```python
from build123d import *

# Parameters (mm, degrees)
SKETCH1_W                                            = 15
SKETCH1_H                                            = 15
SKETCH1_W_2                                          = 4
SKETCH1_H_2                                          = 4
BOSS_EXTRUDE1_DEPTH                                  = 10
FILLET1_R                                            = 0.5
CBORE_FOR_M1_6_HEXAGON_SOCKET_HEAD_CAP_S_D           = 1.8
CBORE_FOR_M1_6_HEXAGON_SOCKET_HEAD_CAP_S_CBORE_D     = 3.3
CBORE_FOR_M1_6_HEXAGON_SOCKET_HEAD_CAP_S_CBORE_DEPTH = 1.8
M2_TAPPED_HOLE1_AT_2_COUNT                           = 2
M2_TAPPED_HOLE1_AT_2_PITCH                           = 9.5
CHAMFER1_SIZE                                        = 1
CUT_EXTRUDE1_DEPTH                                   = 2
M2_TAPPED_HOLE2_D                                    = 1.6
M2_TAPPED_HOLE2_DEPTH                                = 2
M2_TAPPED_HOLE2_TIP                                  = 0.480688495
SKETCH12_R                                           = 4.5
SKETCH12_R_2                                         = 3
CUT_EXTRUDE2_DEPTH                                   = 2
FILLET2_R                                            = 1
CHAMFER2_SIZE                                        = 1


with BuildPart() as part:
    # Sketch1 → Boss-Extrude1 (new body)
    with BuildSketch(Plane.XY):
        Rectangle(SKETCH1_W, SKETCH1_H)
        Rectangle(SKETCH1_W_2, SKETCH1_H_2, mode=Mode.SUBTRACT)
    extrude(amount=-BOSS_EXTRUDE1_DEPTH)

    # Fillet1
    fillet1_edges = [part.edges().sort_by_distance(p)[0] for p in [
        (2, 2, -5),
        (2, -2, -5),
        (-2, -2, -5),
        (-2, 2, -5),
    ]]
    fillet(fillet1_edges, radius=FILLET1_R)

    # CBORE for M1.6 Hexagon socket head cap screws1 (through all)
    with Locations(Plane(origin=(0, 7.5, 0), x_dir=(1, 0, 0), z_dir=(0, 1, 0))):
        with Locations((0, 5)):
            CounterBoreHole(CBORE_FOR_M1_6_HEXAGON_SOCKET_HEAD_CAP_S_D / 2, CBORE_FOR_M1_6_HEXAGON_SOCKET_HEAD_CAP_S_CBORE_D / 2, CBORE_FOR_M1_6_HEXAGON_SOCKET_HEAD_CAP_S_CBORE_DEPTH)

    # Sketch6 → M2 Tapped Hole1 (revolve, cut)
    with BuildSketch(Plane(origin=(-7.5, 5, -5), x_dir=(0, 0, 1), z_dir=(0, 1, 0))):
        Polygon((0, 0), (0, 5.480688495), (0.8, 5), (0.8, 0), align=None)
    m2_tapped_hole1 = revolve(axis=Axis((-13.85, 5, -5), (1, 0, 0)), mode=Mode.SUBTRACT)

    # M2 Tapped Hole1 at 2: M2 Tapped Hole1 ×2
    with Locations(*[(0, -i * M2_TAPPED_HOLE1_AT_2_PITCH, 0) for i in range(1, M2_TAPPED_HOLE1_AT_2_COUNT)]):
        add(m2_tapped_hole1, mode=Mode.SUBTRACT)

    # Mirror1: M2 Tapped Hole1 across plane
    add(m2_tapped_hole1.mirror(Plane(origin=(0, 0, 0), x_dir=(0, 0, 1), z_dir=(1, 0, 0))), mode=Mode.SUBTRACT)

    # Mirror1 copy 1 sketch → Mirror1 copy 1 (revolve, cut)
    with BuildSketch(Plane(origin=(7.5, -4.5, -5), x_dir=(0, 0, 1), z_dir=(0, 1, 0))):
        Polygon((0, 0), (0, -5.480688495), (0.8, -5), (0.8, 0), align=None)
    revolve(axis=Axis((13.85, -4.5, -5), (1, 0, 0)), mode=Mode.SUBTRACT)

    # Chamfer1
    chamfer1_edges = [part.edges().sort_by_distance(p)[0] for p in [
        (7.5, -7.5, -5),
        (-7.5, -7.5, -5),
    ]]
    chamfer(chamfer1_edges, length=CHAMFER1_SIZE)

    # Sketch8 → Cut-Extrude1 (cut)
    with BuildSketch(Plane(origin=(0, 0, -10), x_dir=(-1, 0, 0), z_dir=(0, 0, -1))):
        with BuildLine():
            ThreePointArc((-5.49078868, 5.818181818), (-5.656854249, 5.656854249), (-5.818181818, 5.49078868))
            ThreePointArc((-5.818181818, 5.49078868), (-5.715871463, 1.956735399), (-2.181818182, 2.059045755))
            ThreePointArc((-2.181818182, 2.059045755), (-2.121320344, 2.121320344), (-2.059045755, 2.181818182))
            ThreePointArc((-2.059045755, 2.181818182), (-1.956735399, 5.715871463), (-5.49078868, 5.818181818))
        make_face()
        with BuildLine():
            ThreePointArc((-5.49078868, -5.818181818), (-5.656854249, -5.656854249), (-5.818181818, -5.49078868))
            ThreePointArc((-5.818181818, -5.49078868), (-5.715871463, -1.956735399), (-2.181818182, -2.059045755))
            ThreePointArc((-2.181818182, -2.059045755), (-2.121320344, -2.121320344), (-2.059045755, -2.181818182))
            ThreePointArc((-2.059045755, -2.181818182), (-1.956735399, -5.715871463), (-5.49078868, -5.818181818))
        make_face()
        with BuildLine():
            ThreePointArc((5.49078868, 5.818181818), (5.656854249, 5.656854249), (5.818181818, 5.49078868))
            ThreePointArc((5.818181818, 5.49078868), (5.715871463, 1.956735399), (2.181818182, 2.059045755))
            ThreePointArc((2.181818182, 2.059045755), (2.121320344, 2.121320344), (2.059045755, 2.181818182))
            ThreePointArc((2.059045755, 2.181818182), (1.956735399, 5.715871463), (5.49078868, 5.818181818))
        make_face()
        with BuildLine():
            ThreePointArc((5.49078868, -5.818181818), (5.656854249, -5.656854249), (5.818181818, -5.49078868))
            ThreePointArc((5.818181818, -5.49078868), (5.715871463, -1.956735399), (2.181818182, -2.059045755))
            ThreePointArc((2.181818182, -2.059045755), (2.121320344, -2.121320344), (2.059045755, -2.181818182))
            ThreePointArc((2.059045755, -2.181818182), (1.956735399, -5.715871463), (5.49078868, -5.818181818))
        make_face()
    extrude(amount=-CUT_EXTRUDE1_DEPTH, mode=Mode.SUBTRACT)

    # M2 Tapped Hole2
    with Locations(Plane(origin=(0, 0, -10), x_dir=(-1, 0, 0), z_dir=(0, 0, -1))):
        with Locations((-6, 0), (0, 6), (6, 0), (0, -6)):
            Hole(M2_TAPPED_HOLE2_D / 2, depth=M2_TAPPED_HOLE2_DEPTH)
            with Locations((0, 0, -(M2_TAPPED_HOLE2_DEPTH + M2_TAPPED_HOLE2_TIP / 2))):  # 118° drill point
                Cone(0, M2_TAPPED_HOLE2_D / 2, M2_TAPPED_HOLE2_TIP, mode=Mode.SUBTRACT)

    # Sketch12 → Cut-Extrude2 (cut)
    with BuildSketch(Plane(origin=(0, 0, -10), x_dir=(-1, 0, 0), z_dir=(0, 0, -1))):
        Circle(SKETCH12_R)
        with Locations(Location((0, 0, 0), (0, 0, 180))):
            Circle(SKETCH12_R_2, mode=Mode.SUBTRACT)
    extrude(amount=-CUT_EXTRUDE2_DEPTH, mode=Mode.SUBTRACT)

    # Fillet2
    fillet2_edges = [part.edges().sort_by_distance(p)[0] for p in [
        (1.294196531, 4.309878808, -9),
        (-1.294196531, 4.309878808, -9),
        (4.309878808, 1.294196531, -9),
        (4.309878808, -1.294196531, -9),
        (-1.294196531, -4.309878808, -9),
        (1.294196531, -4.309878808, -9),
        (-4.309878808, -1.294196531, -9),
        (-4.309878808, 1.294196531, -9),
    ]]
    fillet(fillet2_edges, radius=FILLET2_R)

    # Chamfer2
    chamfer2_edges = [part.edges().sort_by_distance(p)[0] for p in [
        (-7.5, 7.5, -5),
        (7.5, 7.5, -5),
    ]]
    chamfer(chamfer2_edges, length=CHAMFER2_SIZE)


solid = part.part
```
The model under review builds one solid part; all positions refer to its coordinate system, in mm. A direction names the side the tool comes from. Give positions to 0.01 mm unless a question says otherwise; leave off trailing zeros. Write each loop counter-clockwise with the first axis right and the second up, starting at its lowest first coordinate (ties: lowest second). Pieces come first, ordered by that corner, then holes.
(1) Consider section A-A, the plane z = -1. Give the boundary of the cut face in (x, y), and give its area (3 significant figures).
(2) Consider section B-B, the plane x = 4. Give the boundary of the cut face in (y, z).
(3) The part is to be moulded in two halves that separate along Y. For faces 1 (the flat face through (0, 5, -10)), 2 (the conical face through (-5.89, -0.08, -7.6)), 3 (the flat face through (7, 7, -5)), say which applies: released by +Y, released by -Y, zero draft, split by the parting line, or undercut.
(4) Tool access review of faces 4 (the flat face through (0, 2, -3.8)), 5 (the cylindrical face through (-6.46, 3.33, -9.01)), 6 (the cylindrical face through (-0.4, 6.6, -3.4)): name each direction out of +Z, -Z, +X, -X, +Y, -Y from which nothing blocks a thin tool from reaching the whole face with its end or side.
(5) To check wall thickness, follow L1, parallel to Y at x = -5.4, z = -5; L2, parallel to Y at x = -2.5, z = -9.5; L3, parallel to X at y = -1, z = -7.5. State the ranges of each line that lie inside material, in increasing order.
(6) Consider section C-C, the plane y = -2.5. Give the boundary of the cut face in (x, z).
(7) Consider section D-D, the plane z = -8.5. Give the number of separate pieces and of enclosed holes in the cut face, and give its area (3 significant figures).
(8) For P1, Ø1.1, axis at x = 0, z = -5, coming from the +Y side; P2, Ø1.3, axis at x = 0, y = -6, coming from the -Z side; P3, Ø1, axis at x = 0, y = 6, coming from the -Z side; P4, Ø1.4, axis at y = -4.5, z = -5, coming from the +X side, all flat-tipped, find the tip position at first contact; note any pin that passes through.
Returned:
1. outline: (-7.5, -6.5) - (-6.5, -7.5) - (6.5, -7.5) - (7.5, -6.5) - (7.5, 6.5) - (6.5, 7.5) - (-6.5, 7.5) - (-7.5, 6.5) - close; hole (-2, -1.5) arc R0.5 ccw to (-1.5, -2) - (1.5, -2) arc R0.5 ccw to (2, -1.5) - (2, 1.5) arc R0.5 ccw to (1.5, 2) - (-1.5, 2) arc R0.5 ccw to (-2, 1.5) - close
1. area: 207 mm2
2. outline: (-7.5, -10) - (-6.49, -10) - (-6.49, -8) - (6.49, -8) - (6.49, -10) - (7.5, -10) - (7.5, 0) - (-7.5, 0) - close; hole circle Ø1.6 at (-4.5, -5); hole circle Ø1.6 at (5, -5)
3. face 1: zero draft
3. face 2: undercut
3. face 3: released by +Y
4. face 4: +Z, -Z
4. face 5: -Z
4. face 6: +Y
5. L1: y = -7.5 to -5.3, -3.7 to 4.2, 5.8 to 7.5
5. L2: y = -7.5 to -6.15, -1.66 to 1.66, 6.15 to 7.5
5. L3: x = -7.5 to -2, 2 to 7.5
6. outline: (-7.5, -10) - (-6.15, -10) - (-6.15, -8) - (-1.66, -8) - (-1.66, -10) - (1.66, -10) - (1.66, -8) - (6.15, -8) - (6.15, -10) - (7.5, -10) - (7.5, 0) - (-7.5, 0) - close; hole circle Ø1.8 at (0, -5)
7. separate pieces: 2
7. enclosed holes: 6
7. area: 95.8 mm2
8. P1: passes through
8. P2: stops at z = -7.91
8. P3: stops at z = -7.82
8. P4: stops at x = 2.44
